Check sheet for the modelled part. Datum: model origin and axes. Units: mm. A direction names the side the tool comes from. Coordinates: 2 decimals unless noted, no trailing zeros. Loops run counter-clockwise (first coordinate to the right, second up) from the corner with the lowest first, then second, coordinate; pieces in that order, holes last. Notation, with made-up numbers: M -20.75,-20 L 6.25,-20 A32 ccw 6.25,10 Z; hole C 41.5,76.5 d11. An arc over 180 degrees is marked long. Write each question's results on one line, items separated by ' | '. Start each with the question number.
from build123d import *

# Parameters (mm, degrees)
EXTRUDE1_DEPTH  = 30
EXTRUDE2_REACH  = 136.629
SKETCH2_R       = 12.5
LPATTERN1_COUNT = 3
LPATTERN1_PITCH = 30


with BuildPart() as part:
    # Sketch1 → Extrude1 (new body)
    with BuildSketch(Plane.XY):
        Polygon((0, 0), (100, -30), (100, 55), (0, 55), align=None)
    extrude(amount=EXTRUDE1_DEPTH)

    # Extrude2: up to this plane
    extrude2_end = Plane(origin=(2.873478856, 9.578262852, 30), z_dir=(0.2873478855663455, 0.9578262852211514, 0))
    # Sketch2 → Extrude2 (cut, up to the surface)
    with BuildSketch(Plane(origin=(0, 55, 0), x_dir=(1, 0, 0), z_dir=(0, 1, 0)), mode=Mode.PRIVATE) as extrude2_sk1:
        with Locations((20, -30)):
            Circle(SKETCH2_R)
    extrude2_tool1 = split(extrude(extrude2_sk1.sketch, amount=-EXTRUDE2_REACH, mode=Mode.PRIVATE), bisect_by=extrude2_end, keep=Keep.BOTH, mode=Mode.PRIVATE)
    extrude2 = extrude2_tool1.solids().sort_by_distance((20, 55, 30))[0]
    add(extrude2, mode=Mode.SUBTRACT)

    # LPattern1: Extrude2 ×3
    with Locations(*[(i * LPATTERN1_PITCH, 0, 0) for i in range(1, LPATTERN1_COUNT)]):
        add(extrude2, mode=Mode.SUBTRACT)


solid = part.part
Item 1: Depth check by flat-ended pin: P1, Ø6, axis at y = 23, z = 5.5, coming from the -X side; P2, Ø3, axis at x = 29, z = 19.5, coming from the -Y side. Enter the tip coordinate at first touch or a pass-through.
Item 2: Tool access check on faces 1 (the face through (19.8, 4.5, 25.1)), 2 (the face through (100, 12, 15)). Record the directions out of +Z, -Z, +X, -X, +Y, -Y that give a thin tool (end or side, any length) a straight path to the whole face; none if there is none.
Item 3: Section check D-D (z = 24.5). Record the cut outline in (x, y).
Item 4: Thickness scan on line 1 (X direction, y = 51.5, z = 24); line 2 (X direction, y = 28, z = 21); line 3 (Z direction, x = 69, y = 45). Record the ranges inside material, lowest first.
Item 5: Section check C-C (x = 80). Record the cut outline in (y, z).
Item 6: Section check A-A (y = 40.5). Record the cut outline in (x, z), plus the area to 3 significant figures.
Item 7: Section check B-B (z = 6.5). Record the cut outline in (x, y), plus the area to 3 significant figures.
Computed values:
1) P1: stops at x = 0 | P2: stops at y = -9.15
2) face 1: +Z, +Y | face 2: +Z, -Z, +X, +Y, -Y
3) outline: M 0,0 L 100,-30 L 100,55 L 91.22,55 L 91.22,1.07 L 68.78,7.81 L 68.78,55 L 61.22,55 L 61.22,1.07 L 38.78,7.81 L 38.78,55 L 31.22,55 L 31.22,1.07 L 8.78,7.81 L 8.78,55 L 0,55 Z
4) line 1: x = 0 to 9.03, 30.97 to 39.03, 60.97 to 69.03, 90.97 to 100 | line 2: x = 0 to 11.33, 28.67 to 41.33, 58.67 to 71.33, 88.67 to 100 | line 3: z = 0 to 24.06
5) outline: M -24,0 L 55,0 L 55,17.5 L 4.44,17.5 L 4.44,30 L -24,30 Z
6) outline: M 0,0 L 100,0 L 100,30 L 92.5,30 A12.5 cw 67.5,30 L 62.5,30 A12.5 cw 37.5,30 L 32.5,30 A12.5 cw 7.5,30 L 0,30 Z | area: 2,260 mm²
7) outline: M 0,0 L 100,-30 L 100,55 L 0,55 Z | area: 7,000 mm²
